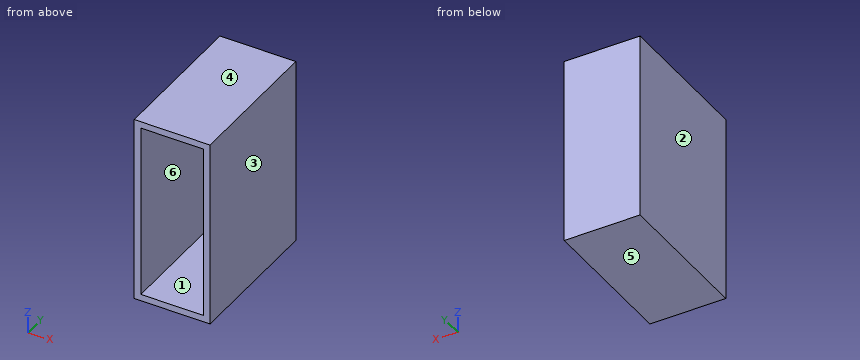
```python
from build123d import *

# Parameters (mm, degrees)
CUBE001_W     = 4.72
CUBE001_H     = 11
CUBE001_DEPTH = 13.2
CUBE_W        = 5.72
CUBE_H        = 11
CUBE_DEPTH    = 14.2


with BuildPart() as cube001:
    # cube001 → cube001 (new body)
    with BuildSketch(Plane(origin=(0.5, -0.5, 0.5), x_dir=(1, 0, 0), z_dir=(0, 0, 1))):
        with Locations((2.36, 5.5)):
            Rectangle(CUBE001_W, CUBE001_H)
    extrude(amount=CUBE001_DEPTH)


with BuildPart() as difference:
    # cube → cube (new body)
    with BuildSketch(Plane.XY):
        with Locations((2.86, 5.5)):
            Rectangle(CUBE_W, CUBE_H)
    extrude(amount=CUBE_DEPTH)

    # difference: cut cube001
    add(cube001.part, mode=Mode.SUBTRACT)


with BuildPart() as difference_1:
    # difference placement: moved
    add(difference.part.moved(Location((-2.86, 0, 0))))


solid = difference_1.part
```
Geometry: final body of the model. Coordinates: model frame, mm. Face numbers are marked on the shaded views. A direction names the side the tool comes from. Round coordinates to 2 decimals unless told otherwise and drop trailing zeros. Loops run counter-clockwise (first coordinate to the right, second up) from the corner with the lowest first, then second, coordinate; pieces in that order, holes last.
Item 1: Section C-C, the plane z = 10.5. Output: boundary loops of the cut face in (x, y), plus the area to 3 significant figures.
Checked values:
outline: (-2.86, 0) - (-2.36, 0) - (-2.36, 10.5) - (2.36, 10.5) - (2.36, 0) - (2.86, 0) - (2.86, 11) - (-2.86, 11) - close
area: 13.4 mm2
Item 2: Section A-A, the plane y = 9.75. Output: boundary loops of the cut face in (x, z).
Checked values:
outline: (-2.86, 0) - (2.86, 0) - (2.86, 14.2) - (-2.86, 14.2) - close; hole (-2.36, 0.5) - (2.36, 0.5) - (2.36, 13.7) - (-2.36, 13.7) - close
Item 3: Section B-B, the plane x = -1.2. Output: boundary loops of the cut face in (y, z).
Checked values:
outline: (0, 0) - (11, 0) - (11, 14.2) - (0, 14.2) - (0, 13.7) - (10.5, 13.7) - (10.5, 0.5) - (0, 0.5) - close
Item 4: Contact query for a flat-ended pin moving along its axis: P1, Ø1.4, axis at x = -1, z = 10, coming from the -Y side. Output: stop coordinate, or through.
Checked values:
P1: stops at y = 10.5
Item 5: Mould query, pull axis X, two halves, no side actions, for the marked faces 1, 2, 3 and 4. Classes: released by +X, released by -X, zero draft, split by the parting line, or undercut.
Checked values:
face 1: undercut
face 2: released by -X
face 3: released by +X
face 4: zero draft
Item 6: Line query: L1, parallel to Z at x = 0.7, y = 2.25; L2, parallel to X at y = 5, z = 1.5; L3, parallel to Y at x = 0.45, z = 9.25. Output: solid intervals per line, ascending.
Checked values:
L1: z = 0 to 0.5, 13.7 to 14.2
L2: x = -2.86 to -2.36, 2.36 to 2.86
L3: y = 10.5 to 11
Item 7: Reachability of the marked faces 5 and 6 from +Z, -Z, +X, -X, +Y, -Y: full face, straight path, thin tool, end or side. Return the list, or none.
Checked values:
face 5: -Z, +X, -X, +Y, -Y
face 6: -Y
